Autodesk Inventor part; units mm, degrees
ref_plane "YZ Plane" through (0, 0, 0) normal (1, 0, 0) x (0, 1, 0)
ref_plane "XZ Plane" through (0, 0, 0) normal (0, 1, 0) x (-1, 0, 0)
ref_plane "XY Plane" through (0, 0, 0) normal (0, 0, 1) x (1, 0, 0)
sketch "Sketch1" plane through (0, 0, 0) normal (0, 1, 0) x (-1, 0, 0)
  line L0 (-3.2, 2.5) -> (3.2, 2.5)
  line L1 (3.2, -2.5) -> (-3.2, -2.5)
  line L2 (-3.2, -2.5) -> (-3.2, 2.5)
  line L3 (-3.2, 2.5) -> (3.2, -2.5) construction
  line L4 (3.2, 2.5) -> (-3.2, -2.5) construction
  circle A0 centre (5.45, 0.0144) radius 2.325
  line L5 (7.7, 2.5) -> (7.7, -2.5)
  line L6 (7.7, -2.5) -> (6.95, -2.5)
  line L7 (6.95, -2.5) -> (6.95, -1.762)
  line L8 (7.7, 2.5) -> (6.95, 2.5)
  line L9 (6.95, 2.5) -> (6.95, 1.7908)
  line L10 (7.7, 2.5) -> (8.7, 2.5)
  line L11 (8.7, 2.5) -> (8.7, -2.5)
  line L12 (8.7, -2.5) -> (7.7, -2.5)
  line L13 (7.7, -2.5) -> (7.7, 2.5)
  line L14 (0, 2.5) -> (0, -2.5)
  line L15 (3.2, -2.5) -> (3.2, 2.5)
  point P0 (0, 0)
  dimension "d1" = 6.4
  dimension "d2" = 5
  dimension "d3" = 4.65
  dimension "d4" = 2.25
  dimension "d5" = 0.75
  dimension "d6" = 1
  dimension "d11" = 2.25
revolve "Revolution1" add sketch "Sketch1" angle 360 about axis through (0, 0, 2.5) along (0, 0, -1) contours L9 L8 L5 A0 | L5 L10 L11 L12 A0 | A0 L5 L6 L7
chamfer "Chamfer1" distance 0.75 angle 45 2 edges at (8.7, 0, -2.5) (8.7, 0, 2.5)
properties part number "5mm Bearing Outside_3DPrint"
Build history of the part. All positions in model axes, mm. Give positions to 0.01 mm unless a question says otherwise; leave off trailing zeros. Order: outer loops, then holes, each group sorted by start corner. A loop starts at its lowest first (then second) coordinate and runs counter-clockwise, first axis right, second up. Notation, with made-up numbers: M 79,63.5 L 133,63.5 A19 ccw 133,94.5 Z; hole C 62.5,-12.75 d11. An arc over 180 degrees is marked long. Write item = value, one per line. Start each with the question number.
(1) Two-plate mould, pull along Y, no slides. Class faces 1 (the cylindrical face through (1.507, 6.785, -2.126)), 2 (the cylindrical face through (1.886, -8.493, -0.024)): released by +Y, released by -Y, zero draft, split by the parting line, or undercut.
(2) Pin check, flat tips, straight feed: pin 1 Ø3 at (y, z) = (4.5, -0.5) entering from +X; pin 2 Ø2 at (y, z) = (-1, 1.5) entering from -X. Stop position of each tip, or through.
(3) Slice it at A-A on y = 0. Write the cut outline in (x, z) (3 decimals).
(4) Slice it at C-C on z = -1.1. Write the cut outline in (x, y).
(5) Probe L1, parallel to X at y = 1.25, z = -2.25; L2, parallel to X at y = 2.75, z = -0.6; L3, parallel to Y at x = 0, z = 2.2. List the from-to ranges inside material, lowest first. Write a range as [from, to].
Responses:
q1.face_1 = undercut
q1.face_2 = split by the parting line
q2.pin_1 = 8.17
q2.pin_2 = -8.7
q3.outline = M -8.7,-1.75 L -7.95,-2.5 L -6.95,-2.5 L -6.95,-1.762 A2.325 cw -6.95,1.791 L -6.95,2.5 L -7.95,2.5 L -8.7,1.75 Z; M 6.95,-2.5 L 7.95,-2.5 L 8.7,-1.75 L 8.7,1.75 L 7.95,2.5 L 6.95,2.5 L 6.95,1.791 A2.325 cw 6.95,-1.762 Z
q4.outline = C 0,0 d17.4; hole C 0,0 d14.98
q5.L1 = [-8.1, -6.84], [6.84, 8.1]
q5.L2 = [-8.25, -7.18], [7.18, 8.25]
q5.L3 = [-8.25, -6.95], [6.95, 8.25]
